```python
from build123d import *

# Parameters (mm, degrees)
F1_DEPTH = 50
F2_R     = 9.5
F3_DEPTH = 177.701
F5_SIZE  = 15
F6_SIZE  = 15


with BuildPart() as f1:
    # F0 (on Front) → F1 (new body)
    with BuildSketch(Plane.XZ):
        Polygon((0, 177.7), (0, 0), (12.7, 0), (12.7, 165), (87.7, 165), (87.7, 0), (100.4, 0), (100.4, 177.7), align=None)
    extrude(amount=F1_DEPTH)

    # F2 (on face) → F3 (cut, through all)
    with BuildSketch(Plane.XY.offset(177.7)):
        with Locations((50.2, -25)):
            Circle(F2_R)
    extrude(amount=-F3_DEPTH, mode=Mode.SUBTRACT)

    # F5
    f5_edges = [f1.edges().sort_by_distance(p)[0] for p in [
        (6.35, -50, 0),
        (6.35, 0, 0),
    ]]
    chamfer(f5_edges, length=F5_SIZE)

    # F6
    f6_edges = [f1.edges().sort_by_distance(p)[0] for p in [
        (94.05, -50, 0),
        (94.05, 0, 0),
    ]]
    chamfer(f6_edges, length=F6_SIZE)


solid = f1.part
```
Model file for the job. Use its own axes, mm. A direction names the side the tool comes from. Coordinates: 2 decimals unless noted, no trailing zeros. Write each loop counter-clockwise with the first axis right and the second up, starting at its lowest first coordinate (ties: lowest second). Pieces come first, ordered by that corner, then holes. Notation, with made-up numbers: (20, -15) - (51, -15) arc R29 ccw to (51, 21) - close; hole circle Ø10 at (86, -8). An arc over 180 degrees is marked (long way). One line per item, written item: value. Start each with the question number.
1. Slice it at A-A (x = 50.2). Write the cut outline in (y, z), plus the area to 3 significant figures.
2. Probe line 1 (X direction, y = -10, z = 64.5); line 2 (Y direction, x = 50.2, z = 170); line 3 (Z direction, x = 60, y = -12). List the from-to ranges inside material, lowest first. Write a range as from..to.
3. Flat gauge pin, fed straight in: pin 1 (1.5 mm diameter, centred on x = 58.5, y = -13, fed in from -Z). Where does the tip first touch, or does it go through?
4. Slice it at B-B (y = -25). Write the cut outline in (x, z), plus the area to 3 significant figures.
5. Mould opens along Y. For faces 1 (the cylindrical face through (59.261, -22.146, 171.439)), 2 (the flat face through (87.7, -25, 84)), 3 (the flat face through (94, -8, 7)), 4 (the flat face through (6, -43, 8)) say: released by +Y, released by -Y, zero draft, split by the parting line, or undercut.
6. Slice it at D-D (y = -47). Write the cut outline in (x, z), plus the area to 3 significant figures.
7. Slice it at C-C (z = 157). Write the cut outline in (x, y).
8. Tool access for faces 5 (the flat face through (0, -25, 90)), 6 (the flat face through (12.7, -25, 81)): list every direction of +Z, -Z, +X, -X, +Y, -Y with a clear straight run to the whole face (end or side of a thin tool).
Answers below:
1. outline: (-50, 165) - (-34.5, 165) - (-34.5, 177.7) - (-50, 177.7) - close; (-15.5, 165) - (0, 165) - (0, 177.7) - (-15.5, 177.7) - close
1. area: 394 mm^2
2. line 1: x = 0..12.7, 87.7..100.4
2. line 2: y = -50..-34.5, -15.5..0
2. line 3: z = 165..177.7
3. pin 1: stops at z = 165
4. outline: (0, 0) - (12.7, 0) - (12.7, 165) - (40.7, 165) - (40.7, 177.7) - (0, 177.7) - close; (59.7, 165) - (87.7, 165) - (87.7, 0) - (100.4, 0) - (100.4, 177.7) - (59.7, 177.7) - close
4. area: 5,220 mm^2
5. face 1: undercut
5. face 2: zero draft
5. face 3: released by +Y
5. face 4: released by -Y
6. outline: (0, 12) - (12.7, 12) - (12.7, 165) - (87.7, 165) - (87.7, 12) - (100.4, 12) - (100.4, 177.7) - (0, 177.7) - close
6. area: 5,160 mm^2
7. outline: (0, -50) - (12.7, -50) - (12.7, 0) - (0, 0) - close; (87.7, -50) - (100.4, -50) - (100.4, 0) - (87.7, 0) - close
8. face 5: +Z, -Z, -X, +Y, -Y
8. face 6: -Z, +Y, -Y
